from build123d import *

# Parameters (mm, degrees)
F0_W     = 360.66404
F0_H     = 159.165882
F1_DEPTH = 33.274
F3_DEPTH = 94.488
F5_D     = 63.5


with BuildPart() as f1:
    # F0 (on Top) → F1 (new body)
    with BuildSketch(Plane.XY):
        Rectangle(F0_W, F0_H)
    extrude(amount=F1_DEPTH)

    # F2 (on Front) → F3 (join)
    with BuildSketch(Plane.XZ):
        Polygon((158.531552, 0), (152.299196, 0), (152.299196, -233.95633), (180.216238, -233.95633), (180.216238, -12.82501), align=None)
    extrude(amount=F3_DEPTH)

    # F5 (through all)
    with Locations(Plane.XY.offset(33.274)):
        with Locations((0, 0)):
            Hole(F5_D / 2)


solid = f1.part
Check sheet for the modelled part. Datum: model origin and axes. Units: mm. A direction names the side the tool comes from. Round coordinates to 2 decimals unless told otherwise and drop trailing zeros. Loops run counter-clockwise (first coordinate to the right, second up) from the corner with the lowest first, then second, coordinate; pieces in that order, holes last.
1. Scan lines: probe 1 along Y at (x, z) = (0, 20.5); probe 2 along X at (y, z) = (-37, -117.5); probe 3 along Z at (x, y) = (-13, 72). Record each from-to range of solid material in increasing order.
2. Gauge pin test, flat ends, axial feed: pin 1 Ø16.5 at (x, z) = (85.5, 9.5) entering from -Y; pin 2 Ø8.5 at (x, z) = (169.5, -160) entering from +Y; pin 3 Ø12 at (y, z) = (-44, -24) entering from -X. Record the tip position at first contact, or that the pin passes through.
3. Mould release check, pull along X, two halves, no side actions. Record for faces 4 (the flat face through (180.216, -47, -125)), 5 (the cylindrical face through (6.883, -30.995, 16.404)), 6 (the flat face through (-3, -79.583, 16)): released by +X, released by -X, zero draft, split by the parting line, or undercut.
4. Sectioned sample at D-D on y = -70.5. Record the boundary of the cut face in (x, z) (3 decimals), and give its area (3 significant figures).
5. Set-up check for faces 1 (the flat face through (152.299, -47, -115)), 2 (the flat face through (166, 0, -115)), 3 (the flat face through (-3, 36, 33.274)): record each of +Z, -Z, +X, -X, +Y, -Y from which the full face is reachable in a straight line by a thin tool's end or side.
6. Sectioned sample at B-B on y = -17. Record the boundary of the cut face in (x, z) (3 decimals), and give its area (3 significant figures).
7. Sectioned sample at A-A on x = 0. Record the boundary of the cut face in (y, z), and give its area (3 significant figures).
8. Sectioned sample at C-C on z = -35.5. Record the boundary of the cut face in (x, y), and give its area (3 significant figures).
Recorded:
1. probe 1: y = -79.58 to -31.75, 31.75 to 79.58
1. probe 2: x = 152.3 to 180.22
1. probe 3: z = 0 to 33.27
2. pin 1: stops at y = -79.58
2. pin 2: stops at y = 0
2. pin 3: stops at x = 152.3
3. face 4: released by +X
3. face 5: undercut
3. face 6: zero draft
4. outline: (-180.332, 0) - (152.299, 0) - (152.299, -233.956) - (180.216, -233.956) - (180.216, -12.825) - (158.532, 0) - (180.332, 0) - (180.332, 33.274) - (-180.332, 33.274) - close
4. area: 18,400 mm2
5. face 1: -Z, -X, +Y, -Y
5. face 2: -Z, +X, -X, +Y
5. face 3: +Z, +X, -X, +Y, -Y
6. outline: (-180.332, 0) - (-26.815, 0) - (-26.815, 33.274) - (-180.332, 33.274) - close; (26.815, 0) - (152.299, 0) - (152.299, -233.956) - (180.216, -233.956) - (180.216, -12.825) - (158.532, 0) - (180.332, 0) - (180.332, 33.274) - (26.815, 33.274) - close
6. area: 16,600 mm2
7. outline: (-79.58, 0) - (-31.75, 0) - (-31.75, 33.27) - (-79.58, 33.27) - close; (31.75, 0) - (79.58, 0) - (79.58, 33.27) - (31.75, 33.27) - close
7. area: 3,180 mm2
8. outline: (152.3, -94.49) - (180.22, -94.49) - (180.22, 0) - (152.3, 0) - close
8. area: 2,640 mm2
